```python
from build123d import *

# Parameters (mm, degrees)
CROQUIS1_W              = 27
CROQUIS1_H              = 14
CROQUIS1_R              = 1.85
SALIENTE_EXTRUIR1_DEPTH = 8
CROQUIS2_W              = 27
CROQUIS2_H              = 6.5
CORTAR_EXTRUIR1_DEPTH   = 5
CROQUIS3_R              = 0.5
SALIENTE_EXTRUIR2_DEPTH = 10


with BuildPart() as part:
    # Croquis1 → Saliente-Extruir1 (new body)
    with BuildSketch(Plane(origin=(0, 0, 0), x_dir=(1, 0, 0), z_dir=(0, 1, 0))):
        with Locations((-13.5, -7)):
            Rectangle(CROQUIS1_W, CROQUIS1_H)
        with Locations(Location((-21.5, -3, 0), (0, 0, 270))):
            Circle(CROQUIS1_R, mode=Mode.SUBTRACT)
        with Locations(Location((-5.5, -3, 0), (0, 0, 90))):
            Circle(CROQUIS1_R, mode=Mode.SUBTRACT)
    extrude(amount=SALIENTE_EXTRUIR1_DEPTH)

    # Croquis2 → Cortar-Extruir1 (cut)
    with BuildSketch(Plane(origin=(0, 8, 0), x_dir=(1, 0, 0), z_dir=(0, 1, 0))):
        with Locations((-13.5, -3.25)):
            Rectangle(CROQUIS2_W, CROQUIS2_H)
    extrude(amount=-CORTAR_EXTRUIR1_DEPTH, mode=Mode.SUBTRACT)

    # Croquis3 → Saliente-Extruir2 (add)
    with BuildSketch(Plane(origin=(0, 0, 0), x_dir=(0, 0, -1), z_dir=(1, 0, 0))):
        with Locations(Location((-13, 1, 0), (0, 0, 180))):
            Circle(CROQUIS3_R)
        with Locations(Location((-11.5, 1, 0), (0, 0, 180))):
            Circle(CROQUIS3_R)
    extrude(amount=SALIENTE_EXTRUIR2_DEPTH)


solid = part.part
```
The model under review builds one solid part; all positions refer to its coordinate system, in mm. A direction names the side the tool comes from. Round coordinates to 2 decimals unless told otherwise and drop trailing zeros. Order: outer loops, then holes, each group sorted by start corner. A loop starts at its lowest first (then second) coordinate and runs counter-clockwise, first axis right, second up. Notation, with made-up numbers: (18, -16) -> (42, -16) arc R20 cw to (42, 18) -> close; hole circle Ø10 at (73, -28). An arc over 180 degrees is marked (long way). Use a Markdown table: item, result.
Q1. Tool access review of faces 1 (the flat face through (-14, 0, 7)), 2 (the cylindrical face through (5, 1, 11)), 3 (the flat face through (-14, 6, 6.5)): name each direction out of +Z, -Z, +X, -X, +Y, -Y from which nothing blocks a thin tool from reaching the whole face with its end or side.
Values:
| item | result |
|---|---|
| face 1 | +Z, -Z, +X, -X, -Y |
| face 2 | +X |
| face 3 | -Z, +X, -X, +Y |
Q2. We need section B-B on y = 1. Write out the cut boundary in (x, z), then the cut area to 3 significant figures.
Values:
| item | result |
|---|---|
| outline | (-27, 0) -> (0, 0) -> (0, 11) -> (10, 11) -> (10, 12) -> (0, 12) -> (0, 12.5) -> (10, 12.5) -> (10, 13.5) -> (0, 13.5) -> (0, 14) -> (-27, 14) -> close; hole circle Ø3.7 at (-21.5, 3); hole circle Ø3.7 at (-5.5, 3) |
| area | 376 mm^2 |
Q3. For line 1 (X direction, y = 2.1, z = 3); line 2 (Z direction, x = -21.5, y = 2); line 3 (Z direction, x = -16, y = 4.75), list the stretches that pass through material, from the lowest coordinate up.
Values:
| item | result |
|---|---|
| line 1 | x = -27 to -23.35, -19.65 to -7.35, -3.65 to 0 |
| line 2 | z = 0 to 1.15, 4.85 to 14 |
| line 3 | z = 6.5 to 14 |
Q4. Mouldability with a two-part tool opening along Z and no side actions: class faces 4 (the flat face through (-14, 4, 14)), 5 (the flat face through (-14, 8, 10)), 6 (the cylindrical face through (-19.666, 1.479, 2.759)) as +Z half, -Z half, draft (parallel to the pull), parting line (faces both ways), or undercut.
Values:
| item | result |
|---|---|
| face 4 | +Z half |
| face 5 | draft |
| face 6 | undercut |
Q5. We need section D-D on z = 13. Write out the cut boundary in (x, y), then the cut area to 3 significant figures.
Values:
| item | result |
|---|---|
| outline | (-27, 0) -> (0, 0) -> (0, 0.5) -> (10, 0.5) -> (10, 1.5) -> (0, 1.5) -> (0, 8) -> (-27, 8) -> close |
| area | 226 mm^2 |
Q6. Clearance check with flat-ended pins moving along their axes: P1, Ø4, axis at y = 1, z = 2, coming from the +X side; P2, Ø3, axis at x = -12.5, z = 2, coming from the +Y side. State where each tip first meets the part, or that it passes through.
Values:
| item | result |
|---|---|
| P1 | stops at x = 0 |
| P2 | stops at y = 3 |
Q7. We need section A-A on z = 3. Write out the cut boundary in (x, y).
Values:
| item | result |
|---|---|
| outline | (-27, 0) -> (-23.35, 0) -> (-23.35, 3) -> (-27, 3) -> close; (-19.65, 0) -> (-7.35, 0) -> (-7.35, 3) -> (-19.65, 3) -> close; (-3.65, 0) -> (0, 0) -> (0, 3) -> (-3.65, 3) -> close |
Q8. We need section C-C on x = -5.5. Write out the cut boundary in (y, z).
Values:
| item | result |
|---|---|
| outline | (0, 0) -> (3, 0) -> (3, 1.15) -> (0, 1.15) -> close; (0, 4.85) -> (3, 4.85) -> (3, 6.5) -> (8, 6.5) -> (8, 14) -> (0, 14) -> close |
